```python
from build123d import *

# Parameters (mm, degrees)
SKETCH2_R                = 0.6
BOSS_EXTRUDE1_DEPTH      = 0.5
SKETCH3_R                = 0.6
BOSS_EXTRUDE2_DEPTH      = 2
BOSS_EXTRUDE2_DEPTH_BACK = 0.5


with BuildPart() as part:
    # Sketch2 → Boss-Extrude1 (new body)
    with BuildSketch(Plane.XY):
        with BuildLine():
            Line((-1.395963948, 1.75), (2.515834251, 1.75))
            ThreePointArc((2.515834251, 1.75), (4.137889568, 0.656838298), (3.733466312, -1.256929657))
            Line((3.733466312, -1.256929657), (2.257187702, -2.687052781))
            ThreePointArc((2.257187702, -2.687052781), (1.620755288, -3.363652659), (1.049849305, -4.096387243))
            ThreePointArc((1.049849305, -4.096387243), (0.559935151, -4.35), (0.070020998, -4.096387243))
            ThreePointArc((0.070020998, -4.096387243), (-0.500884985, -3.363652659), (-1.137317399, -2.687052781))
            Line((-1.137317399, -2.687052781), (-2.61359601, -1.256929657))
            ThreePointArc((-2.61359601, -1.256929657), (-3.018019265, 0.656838298), (-1.395963948, 1.75))
        make_face()
        with Locations((-1.395963948, 0)):
            Circle(SKETCH2_R, mode=Mode.SUBTRACT)
        with Locations((2.515834251, 0)):
            Circle(SKETCH2_R, mode=Mode.SUBTRACT)
    extrude(amount=BOSS_EXTRUDE1_DEPTH)

    # Sketch3 → Boss-Extrude2 (add, two sides)
    with BuildSketch(Plane.XY.offset(0.5)) as boss_extrude2_sk:
        with Locations((-1.395963948, 0)):
            Circle(SKETCH3_R)
        with Locations((2.515834251, 0)):
            Circle(SKETCH3_R)
    extrude(amount=BOSS_EXTRUDE2_DEPTH)
    extrude(boss_extrude2_sk.sketch, amount=-BOSS_EXTRUDE2_DEPTH_BACK)


solid = part.part
```
Can you work these out from the model? Positions are in its coordinate system, mm. A direction names the side the tool comes from. Coordinates: 2 decimals unless noted, no trailing zeros. Loops run counter-clockwise (first coordinate to the right, second up) from the corner with the lowest first, then second, coordinate; pieces in that order, holes last. Notation, with made-up numbers: (-4, 43) - (34, 43) arc R27 ccw to (34, 67) - close; hole circle Ø2 at (16.25, 56.25). An arc over 180 degrees is marked (long way). Use a Markdown table: item, result.
Item 1: We'd pull the mould along X, two halves only. Please class faces 3 (the face through (2.5, 0, 2.5)), 4 (the face through (-0.492, -3.374, 0.246)), 5 (the face through (1.916, 0.026, 1.486)): released by +X, released by -X, zero draft, split by the parting line, or undercut.
Numbers:
| item | result |
|---|---|
| face 3 | zero draft |
| face 4 | released by -X |
| face 5 | undercut |
Item 2: I want a section at A-A on z = 1.95. Please give me the cut outline in (x, y), and give its area (3 significant figures).
Numbers:
| item | result |
|---|---|
| outline | circle Ø1.2 at (-1.4, 0); circle Ø1.2 at (2.52, 0) |
| area | 2.26 mm2 |
Item 3: I want a section at D-D on x = -2.25. Please give me the cut outline in (y, z).
Numbers:
| item | result |
|---|---|
| outline | (-1.61, 0) - (1.53, 0) - (1.53, 0.5) - (-1.61, 0.5) - close |
Item 4: I want a section at C-C on z = 0.4. Please give me the cut outline in (x, y).
Numbers:
| item | result |
|---|---|
| outline | (-2.61, -1.26) - (-1.14, -2.69) arc R10 cw to (0.07, -4.1) arc R0.6 ccw to (1.05, -4.1) arc R10 cw to (2.26, -2.69) - (3.73, -1.26) arc R1.75 ccw to (2.52, 1.75) - (-1.4, 1.75) arc R1.75 ccw to start |
Item 5: I want a section at B-B on y = 0. Please give me the cut outline in (x, z).
Numbers:
| item | result |
|---|---|
| outline | (-3.15, 0) - (4.27, 0) - (4.27, 0.5) - (3.12, 0.5) - (3.12, 2.5) - (1.92, 2.5) - (1.92, 0.5) - (-0.8, 0.5) - (-0.8, 2.5) - (-2, 2.5) - (-2, 0.5) - (-3.15, 0.5) - close |
Item 6: For faces 1 (the face through (4.13, 0.68, 0.25)), 2 (the face through (1, -1, 0.5)), which set-ups out of +Z, -Z, +X, -X, +Y, -Y let a thin tool reach every point of the face, with its end or its side?
Numbers:
| item | result |
|---|---|
| face 1 | +Z, -Z, +X |
| face 2 | +Z |
Item 7: If I drill on probe 1 along Z at (x, y) = (0.5, -1); probe 2 along X at (y, z) = (0.5, 1.1); probe 3 along X at (y, z) = (0.25, 1.75), over which ranges is the centre line in solid material (lowest first)? Write a range as from..to.
Numbers:
| item | result |
|---|---|
| probe 1 | z = 0..0.5 |
| probe 2 | x = -1.73..-1.06, 2.18..2.85 |
| probe 3 | x = -1.94..-0.85, 1.97..3.06 |
